Can you work these out from the model? Positions are in its coordinate system, mm. Face numbers are marked on the shaded views. A direction names the side the tool comes from. Give positions to 0.01 mm unless a question says otherwise; leave off trailing zeros. Loops run counter-clockwise (first coordinate to the right, second up) from the corner with the lowest first, then second, coordinate; pieces in that order, holes last.
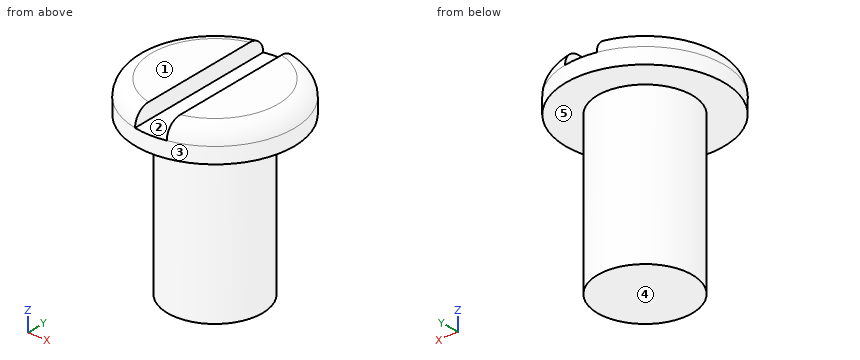
Solid Edge part; units mm, degrees
sketch "Sketch1" plane through (0, 0, 0) normal (0, 0, 1) x (1, 0, 0)
  circle A0 centre (0, 0) radius 1.5
extrude "Protrusion1" add sketch "Sketch1" along normal blind 5
sketch "Sketch2" plane through (0, 0, 5) normal (0, 0, 1) x (1, 0, 0)
  circle A0 centre (0, 0) radius 2.5
extrude "Head" add sketch "Sketch2" along normal blind 1
fillet "Round___Head" radius 0.5 1 edges at (-2.5, 0, 6)
sketch "Sketch3" plane through (0, 0, 6) normal (0, 0, 1) x (1, 0, 0)
  line L0 (-0.5, -2.4495) -> (-0.5, 2.4495)
  line L1 (0.5, 2.4495) -> (0.5, -2.4495)
  arc A0 (0.5, -2.4495) -> (-0.5, -2.4495) centre (0, 0) cw
  arc A1 (-0.5, 2.4495) -> (0.5, 2.4495) centre (0, 0) cw
extrude "Cutout___Head" cut sketch "Sketch3" against normal blind 0.5
cosmetic_thread "Thread1"
properties material "Stainless Steel, 420"
(1) Please list where these lines run through material, in increasing order: probe 1 along Z at (x, y) = (-0.2, -0.9); probe 2 along Z at (x, y) = (0.1, 1.7); probe 3 along X at (y, z) = (-1, 1).
Returned:
probe 1: z = 0 to 5.5
probe 2: z = 5 to 5.5
probe 3: x = -1.12 to 1.12
(2) Which directions (+Z, -Z, +X, -X, +Y, -Y) give clear straight access to the entire face, cutting with the end or side of a thin tool? Please do the marked faces 4 and 5.
Returned:
face 4: -Z, +X, -X, +Y, -Y
face 5: -Z
(3) Thinking about a two-plate mould opening in X: for the marked faces 1, 2 and 3, which applies, pulls with the +X half, pulls with the -X half, needs draft (parallel to the pull), parting line crosses it, or undercut?
Returned:
face 1: needs draft
face 2: undercut
face 3: parting line crosses it
(4) Will these pins go through, and if not, where does the flat tip stop? P1, Ø1.1, axis at x = 0, y = 0, coming from the +Z side; P2, Ø1, axis at y = -0.5, z = 3.5, coming from the +X side; P3, Ø2, axis at y = 1.5, z = 1.5, coming from the -X side; P4, Ø2, axis at x = -2, z = 2.5, coming from the +Y side.
Returned:
P1: stops at z = 6
P2: stops at x = 1.5
P3: stops at x = -1.41
P4: stops at y = 1.12
(5) Suppose I cut it at A-A on x = 0. List the corners of the cut face in (y, z) for me, plus the area to 3 significant figures.
Returned:
outline: (-2.5, 5) - (-1.5, 5) - (-1.5, 0) - (1.5, 0) - (1.5, 5) - (2.5, 5) - (2.5, 5.5) - (-2.5, 5.5) - close
area: 17.5 mm2
(6) Suppose I cut it at C-C on z = 1. List the corners of the cut face in (x, y) for me, plus the area to 3 significant figures.
Returned:
outline: circle Ø3 at (0, 0)
area: 7.07 mm2
(7) Suppose I cut it at B-B on y = 0. List the corners of the cut face in (x, z) for me, plus the area to 3 significant figures.
Returned:
outline: (-2.5, 5) - (-1.5, 5) - (-1.5, 0) - (1.5, 0) - (1.5, 5) - (2.5, 5) - (2.5, 5.5) arc R0.5 ccw to (2, 6) - (0.5, 6) - (0.5, 5.5) - (-0.5, 5.5) - (-0.5, 6) - (-2, 6) arc R0.5 ccw to (-2.5, 5.5) - close
area: 19.4 mm2
